```python
from build123d import *

# Parameters (mm, degrees)
F0_R     = 34.280091
F1_DEPTH = 40
F3_DEPTH = 25
F5_DEPTH = 25


with BuildPart() as f1:
    # F0 (on Top) → F1 (new body)
    with BuildSketch(Plane.XY):
        with Locations((-24.425134, 29.899733)):
            Circle(F0_R)
    extrude(amount=F1_DEPTH)

    # F2 (on face) → F3 (cut)
    with BuildSketch(Plane.XY.offset(40)):
        with BuildLine():
            ThreePointArc((-13.213922, 62.294692), (-24.425134, 64.179824), (-35.636346, 62.294692))
            ThreePointArc((-35.636346, 62.294692), (-24.425134, 56.870885), (-13.213922, 62.294692))
        make_face()
        with BuildLine():
            ThreePointArc((-13.213922, 62.294692), (-10.920198, 66.471352), (-10.126233, 71.169786))
            ThreePointArc((-10.126233, 71.169786), (-29.123568, 84.674722), (-35.636346, 62.294692))
            ThreePointArc((-35.636346, 62.294692), (-24.425134, 64.179824), (-13.213922, 62.294692))
        make_face()
        with BuildLine():
            ThreePointArc((9.854957, 29.899733), (8.074967, 40.802397), (2.919848, 50.572822))
            ThreePointArc((2.919848, 50.572822), (1.225956, 38.234277), (9.848758, 29.24783))
            ThreePointArc((9.848758, 29.24783), (9.853407, 29.573767), (9.854957, 29.899733))
        make_face()
        with BuildLine():
            ThreePointArc((29.12392, 42.652881), (18.961908, 56.340274), (2.919848, 50.572822))
            ThreePointArc((2.919848, 50.572822), (8.074967, 40.802397), (9.854957, 29.899733))
            ThreePointArc((9.854957, 29.899733), (9.853407, 29.573767), (9.848758, 29.24783))
            ThreePointArc((9.848758, 29.24783), (22.989071, 30.913766), (29.12392, 42.652881))
        make_face()
        with BuildLine():
            ThreePointArc((14.131696, -3.488441), (11.224856, 5.15329), (3.686206, 10.281446))
            ThreePointArc((3.686206, 10.281446), (-4.275802, 2.166557), (-14.453916, -2.898124))
            ThreePointArc((-14.453916, -2.898124), (-0.462427, -17.784294), (14.131696, -3.488441))
        make_face()
        with BuildLine():
            ThreePointArc((-14.453916, -2.898124), (-4.275802, 2.166557), (3.686206, 10.281446))
            ThreePointArc((3.686206, 10.281446), (-8.571889, 8.079613), (-14.453916, -2.898124))
        make_face()
        with BuildLine():
            ThreePointArc((-34.396352, -2.898124), (-40.278379, 8.079613), (-52.536474, 10.281446))
            ThreePointArc((-52.536474, 10.281446), (-44.574466, 2.166557), (-34.396352, -2.898124))
        make_face()
        with BuildLine():
            ThreePointArc((-34.396352, -2.898124), (-44.574466, 2.166557), (-52.536474, 10.281446))
            ThreePointArc((-52.536474, 10.281446), (-57.324793, -14.880502), (-34.384161, -3.488441))
            ThreePointArc((-34.384161, -3.488441), (-34.387209, -3.19322), (-34.396352, -2.898124))
        make_face()
        with BuildLine():
            ThreePointArc((-58.699026, 29.24783), (-57.027438, 40.492864), (-51.770116, 50.572822))
            ThreePointArc((-51.770116, 50.572822), (-77.27435, 47.071485), (-58.699026, 29.24783))
        make_face()
        with BuildLine():
            ThreePointArc((-49.376386, 42.652881), (-49.987894, 46.78977), (-51.770116, 50.572822))
            ThreePointArc((-51.770116, 50.572822), (-57.027438, 40.492864), (-58.699026, 29.24783))
            ThreePointArc((-58.699026, 29.24783), (-51.936172, 34.488828), (-49.376386, 42.652881))
        make_face()
    extrude(amount=-F3_DEPTH, mode=Mode.SUBTRACT)

    # F4 (on face) → F5 (cut)
    with BuildSketch(Plane(origin=(0, 0, 0), x_dir=(1, 0, 0), z_dir=(0, 0, -1))):
        Polygon((-24.329751, -35.569776), (-19.467041, -32.652151), (-19.562424, -26.982108), (-24.520517, -24.22969), (-29.383227, -27.147316), (-29.287844, -32.817359), align=None)
    extrude(amount=-F5_DEPTH, mode=Mode.SUBTRACT)


solid = f1.part
```
Verification items for the finished model (mm, model axes). A direction names the side the tool comes from. Give positions to 0.01 mm unless a question says otherwise; leave off trailing zeros. Order: outer loops, then holes, each group sorted by start corner. A loop starts at its lowest first (then second) coordinate and runs counter-clockwise, first axis right, second up. Notation, with made-up numbers: (5.5, 39.5) -> (47.5, 39.5) arc R30 cw to (47.5, 67.5) -> close; hole circle Ø6 at (-38, 52). An arc over 180 degrees is marked (long way). One line per item, written item: value.
(1) Sectioned sample at B-B on z = 12. Record the cut outline in (x, y).
Final values:
outline: circle Ø68.56 at (-24.43, 29.9); hole (-29.38, 27.15) -> (-24.52, 24.23) -> (-19.56, 26.98) -> (-19.47, 32.65) -> (-24.33, 35.57) -> (-29.29, 32.82) -> close
(2) Tool access check on faces 5 (the face through (-21.93, 34.13, 12.32)), 6 (the face through (-25, 61, 15)), 7 (the face through (-40.13, 7.97, 27.68)), 8 (the face through (1.17, 38.41, 27.68)). Record the directions out of +Z, -Z, +X, -X, +Y, -Y that give a thin tool (end or side, any length) a straight path to the whole face; none if there is none.
Final values:
face 5: -Z
face 6: +Z, +Y
face 7: +Z, -Y
face 8: +Z, +X
(3) Scan lines: line 1 along Z through (x, y) = (-34, 61.5); line 2 along X through (y, z) = (34.5, 21); line 3 along X through (y, z) = (27.5, 7). Record each from-to range of solid material in increasing order. Write a range as [from, to].
Final values:
line 1: [0, 15]
line 2: [-51.93, -26.26], [-22.55, 3.08]
line 3: [-58.62, -29.38], [-19.55, 9.77]
(4) Sectioned sample at C-C on x = -46. Record the cut outline in (y, z), then the cut area to 3 significant figures.
Final values:
outline: (3.26, 0) -> (56.54, 0) -> (56.54, 40) -> (10.56, 40) -> (10.56, 15) -> (3.26, 15) -> close
area: 1,950 mm^2
(5) Sectioned sample at A-A on y = 5. Record the cut outline in (x, z).
Final values:
outline: (-47.99, 0) -> (-0.86, 0) -> (-0.86, 15) -> (-11.67, 15) -> (-11.67, 40) -> (-37.18, 40) -> (-37.18, 15) -> (-47.99, 15) -> close
(6) Gauge pin test, flat ends, axial feed: pin 1 (4 mm diameter, centred on x = -25.5, z = 4, fed in from -Y); pin 2 (4 mm diameter, centred on x = -40, z = 26.5, fed in from -Y); pin 3 (3 mm diameter, centred on x = -55.5, y = 35, fed in from +Z). Record the tip position at first contact, or that the pin passes through.
Final values:
pin 1: y = -4.38
pin 2: y = 6.02
pin 3: z = 15
(7) Draft check along X on faces 1 (the face through (8.27, 40.2, 10.83)), 2 (the face through (5, 40, 15)), 3 (the face through (-24, 30, 25)), 4 (the face through (-8.43, 8.18, 27.68)). Enter one of: pulls with the +X half, pulls with the -X half, needs draft (parallel to the pull), parting line crosses it, or undercut.
Final values:
face 1: parting line crosses it
face 2: needs draft
face 3: undercut
face 4: undercut
(8) Sectioned sample at D-D on z = 30. Record the cut outline in (x, y).
Final values:
outline: (-58.7, 29.25) arc R34.28 ccw to (-52.54, 10.28) arc R14.3 cw to (-34.4, -2.9) arc R34.28 ccw to (-14.45, -2.9) arc R14.3 cw to (3.69, 10.28) arc R34.28 ccw to (9.85, 29.25) arc R14.3 cw to (2.92, 50.57) arc R34.28 ccw to (-13.21, 62.29) arc R14.3 cw to (-35.64, 62.29) arc R34.28 ccw to (-51.77, 50.57) arc R14.3 cw to (-49.38, 42.65) arc R14.3 cw to start
